Here's how the part is built. I have some questions about the finished solid (model axes, mm). A direction names the side the tool comes from. Round coordinates to 2 decimals unless told otherwise and drop trailing zeros. Order: outer loops, then holes, each group sorted by start corner. A loop starts at its lowest first (then second) coordinate and runs counter-clockwise, first axis right, second up. Notation, with made-up numbers: (-1.5, -25) -> (47.5, -25) arc R14 cw to (47.5, -8) -> close; hole circle Ø2 at (53, -8). An arc over 180 degrees is marked (long way). Use a Markdown table: item, result. Add a question column.
from build123d import *

# Parameters (mm, degrees)
CROQUIS2_W              = 150
CROQUIS2_H              = 150
CROQUIS2_W_2            = 99.2
CROQUIS2_H_2            = 99.2
SALIENTE_EXTRUIR1_DEPTH = 3
CROQUIS5_W              = 150
CROQUIS5_H              = 150
CROQUIS5_W_2            = 144
CROQUIS5_H_2            = 144
SALIENTE_EXTRUIR2_DEPTH = 25.4
CROQUIS6_R              = 3.175
SALIENTE_EXTRUIR3_DEPTH = 15


with BuildPart() as part:
    # Croquis2 → Saliente-Extruir1 (new body)
    with BuildSketch(Plane.XY):
        Rectangle(CROQUIS2_W, CROQUIS2_H)
        Rectangle(CROQUIS2_W_2, CROQUIS2_H_2, mode=Mode.SUBTRACT)
    extrude(amount=SALIENTE_EXTRUIR1_DEPTH)

    # Croquis5 → Saliente-Extruir2 (add)
    with BuildSketch(Plane.XY.offset(3)):
        Rectangle(CROQUIS5_W, CROQUIS5_H)
        Rectangle(CROQUIS5_W_2, CROQUIS5_H_2, mode=Mode.SUBTRACT)
    extrude(amount=SALIENTE_EXTRUIR2_DEPTH)

    # Croquis6 → Saliente-Extruir3 (add)
    with BuildSketch(Plane(origin=(0, 0, 0), x_dir=(-1, 0, 0), z_dir=(0, 0, -1))):
        with Locations(Location((31.07, -55.9, 0), (0, 0, 180))):
            Circle(CROQUIS6_R)
    extrude(amount=SALIENTE_EXTRUIR3_DEPTH)


solid = part.part
(1) I want a section at D-D on y = 56. List the corners of the cut face in (x, z) for me, and give its area (3 significant figures).
(2) I'm going to push flat-ended pins straight in: P1, Ø8, axis at x = -30, z = -10, coming from the +Y side (3 decimals); P2, Ø1.5, axis at x = -15, y = -52.5, coming from the +Z side. Where does each tip first touch, or does it pass through?
(3) I want a section at C-C on y = -45.5. List the corners of the cut face in (x, z) for me.
(4) On a 3-axis mill with a long thin cutter (end or side, diameter ignored), from which of +Z, -Z, +X, -X, +Y, -Y can I reach the whole of each face in a straight line? I mean faces 5 (the flat face through (-1, -75, 14)), 6 (the cylindrical face through (-31.76, -52.8, -7.4)), 7 (the flat face through (72, -1, 16)). Say none if no direction works.
(5) I want a section at B-B on z = 7. List the corners of the cut face in (x, y) for me.
(6) Please list where these lines run through material, in increasing order: probe 1 along X at (y, z) = (-31, 4.5); probe 2 along X at (y, z) = (0.5, 1.5). Write a range as from..to.
(7) If we mould it in two halves opening along X, with no side actions, what happens to faces 1 (the flat face through (-1, -72, 16)), 2 (the flat face through (-72, -1, 16)), 3 (the flat face through (-75, -1, 14)), 4 (the flat face through (-31, -56, -15))? For each: pulls with the +X half, pulls with the -X half, needs draft (parallel to the pull), parting line crosses it, or undercut.
(8) I want a section at A-A on x = -31.07. List the corners of the cut face in (y, z) for me (3 decimals).
Output:
| question | item | result |
|---|---|---|
| 1 | outline | (-75, 0) -> (75, 0) -> (75, 28.4) -> (72, 28.4) -> (72, 3) -> (-72, 3) -> (-72, 28.4) -> (-75, 28.4) -> close |
| 1 | area | 602 mm² |
| 2 | P1 | y = -52.725 |
| 2 | P2 | z = 3 |
| 3 | outline | (-75, 0) -> (-49.6, 0) -> (-49.6, 3) -> (-72, 3) -> (-72, 28.4) -> (-75, 28.4) -> close; (49.6, 0) -> (75, 0) -> (75, 28.4) -> (72, 28.4) -> (72, 3) -> (49.6, 3) -> close |
| 4 | face 5 | +Z, -Z, +X, -X, -Y |
| 4 | face 6 | -Z |
| 4 | face 7 | +Z |
| 5 | outline | (-75, -75) -> (75, -75) -> (75, 75) -> (-75, 75) -> close; hole (-72, -72) -> (72, -72) -> (72, 72) -> (-72, 72) -> close |
| 6 | probe 1 | -75..-72, 72..75 |
| 6 | probe 2 | -75..-49.6, 49.6..75 |
| 7 | face 1 | undercut |
| 7 | face 2 | undercut |
| 7 | face 3 | pulls with the -X half |
| 7 | face 4 | needs draft |
| 8 | outline | (-75, 0) -> (-59.075, 0) -> (-59.075, -15) -> (-52.725, -15) -> (-52.725, 0) -> (-49.6, 0) -> (-49.6, 3) -> (-72, 3) -> (-72, 28.4) -> (-75, 28.4) -> close; (49.6, 0) -> (75, 0) -> (75, 28.4) -> (72, 28.4) -> (72, 3) -> (49.6, 3) -> close |
